The model under review builds one solid part; all positions refer to its coordinate system, in mm. A direction names the side the tool comes from. Round coordinates to 2 decimals unless told otherwise and drop trailing zeros. Loops run counter-clockwise (first coordinate to the right, second up) from the corner with the lowest first, then second, coordinate; pieces in that order, holes last. Notation, with made-up numbers: (80, 22) -> (136, 22) arc R26 ccw to (136, 46) -> close; hole circle Ø6 at (-14, -30.75). An arc over 180 degrees is marked (long way). Use CSV: the item, a comma, the result in double quotes. Start each with the question number.
```python
from build123d import *

# Parameters (mm, degrees)
CROQUIS1_R                        = 13.5
SALIENTE_EXTRUIR1_DEPTH           = 6
CROQUIS3_R                        = 1.575
CORTAR_EXTRUIR1_DEPTH             = 1.8
DI_METRO_DE_TALADRO_3_0_3_2_D     = 3
DI_METRO_DE_TALADRO_3_0_3_2_DEPTH = 50
DI_METRO_DE_TALADRO_3_0_3_2_TIP   = 0.901290929


with BuildPart() as part:
    # Croquis1 → Saliente-Extruir1 (new body)
    with BuildSketch(Plane.XY):
        Circle(CROQUIS1_R)
    extrude(amount=SALIENTE_EXTRUIR1_DEPTH)

    # Croquis3 → Cortar-Extruir1 (cut)
    with BuildSketch(Plane(origin=(0, 0, 0), x_dir=(-1, 0, 0), z_dir=(0, 0, -1))):
        with Locations((10.5, 0)):
            Circle(CROQUIS3_R)
        with Locations((-7.5, 0)):
            Circle(CROQUIS3_R)
    extrude(amount=-CORTAR_EXTRUIR1_DEPTH, mode=Mode.SUBTRACT)

    # Diámetro de taladro Ø3.0 (3)2
    with Locations(Plane.XY.offset(6)):
        with Locations((-4.949747468, 4.949747468), (-4.949747468, -4.949747468), (4.949747468, -4.949747468), (4.949747468, 4.949747468)):
            Hole(DI_METRO_DE_TALADRO_3_0_3_2_D / 2, depth=DI_METRO_DE_TALADRO_3_0_3_2_DEPTH)
            with Locations((0, 0, -(DI_METRO_DE_TALADRO_3_0_3_2_DEPTH + DI_METRO_DE_TALADRO_3_0_3_2_TIP / 2))):  # 118° drill point
                Cone(0, DI_METRO_DE_TALADRO_3_0_3_2_D / 2, DI_METRO_DE_TALADRO_3_0_3_2_TIP, mode=Mode.SUBTRACT)


solid = part.part
```
1. Clearance check with flat-ended pins moving along their axes: P1, Ø1, axis at y = 3.5, z = 1.5, coming from the +X side; P2, Ø3, axis at y = -2.5, z = 1.5, coming from the -X side; P3, Ø1.6, axis at x = -11, y = -0.5, coming from the -Z side. State where each tip first meets the part, or that it passes through.
2. Take a section at D-D, the plane x = -10.5. Give the boundary of the cut face in (y, z) (3 decimals), then the cut area to 3 significant figures.
3. Take a section at A-A, the plane y = 0. Give the boundary of the cut face in (x, z) (3 decimals), then the cut area to 3 significant figures.
4. The part is to be moulded in two halves that separate along X. For faces 1 (the face through (9.073, 0.069, 0.887)), 2 (the face through (0, 0, 6)), 3 (the face through (-2.93, -13.18, 2.96)), say which applies: pulls with the +X half, pulls with the -X half, needs draft (parallel to the pull), parting line crosses it, or undercut.
5. Take a section at C-C, the plane x = 7.5. Give the boundary of the cut face in (y, z) (3 decimals).
6. Take a section at B-B, the plane y = -5.5. Give the boundary of the cut face in (x, z), then the cut area to 3 significant figures.
7. For line 1 along Y through (x, z) = (-4.25, 2.05); line 2 along X through (y, z) = (4.75, 4.15); line 3 along X through (y, z) = (0.25, 2.65), list the stretches that pass through material, from the lowest coordinate up. Write a range as from..to.
8. For faces 4 (the face through (8, 0, 1.8)), 5 (the face through (-5.756, -3.685, 2.958)), list the 3-axis set-ups (+Z, -Z, +X, -X, +Y, -Y) from which the entire face can be reached by the end or side of a thin tool; tool diameter is ignored.
Results:
1,P1,"x = 13.16"
1,P2,"x = -13.46"
1,P3,"z = 1.8"
2,outline,"(-8.485, 0) -> (-1.575, 0) -> (-1.575, 1.8) -> (1.575, 1.8) -> (1.575, 0) -> (8.485, 0) -> (8.485, 6) -> (-8.485, 6) -> close"
2,area,"96.2 mm²"
3,outline,"(-13.5, 0) -> (-12.075, 0) -> (-12.075, 1.8) -> (-8.925, 1.8) -> (-8.925, 0) -> (5.925, 0) -> (5.925, 1.8) -> (9.075, 1.8) -> (9.075, 0) -> (13.5, 0) -> (13.5, 6) -> (-13.5, 6) -> close"
3,area,"151 mm²"
4,face 1,"undercut"
4,face 2,"needs draft"
4,face 3,"parting line crosses it"
5,outline,"(-11.225, 0) -> (-1.575, 0) -> (-1.575, 1.8) -> (1.575, 1.8) -> (1.575, 0) -> (11.225, 0) -> (11.225, 6) -> (-11.225, 6) -> close"
6,outline,"(-12.33, 0) -> (-6.35, 0) -> (-6.35, 6) -> (-12.33, 6) -> close; (-3.55, 0) -> (3.55, 0) -> (3.55, 6) -> (-3.55, 6) -> close; (6.35, 0) -> (12.33, 0) -> (12.33, 6) -> (6.35, 6) -> close"
6,area,"114 mm²"
7,line 1,"-12.81..-6.28, -3.62..3.62, 6.28..12.81"
7,line 2,"-12.64..-6.44, -3.46..3.46, 6.44..12.64"
7,line 3,"-13.5..13.5"
8,face 4,"-Z"
8,face 5,"+Z, -Z"
